Autodesk Inventor part; units mm, degrees
ref_plane "YZ Plane" through (0, 0, 0) normal (1, 0, 0) x (0, 1, 0)
ref_plane "XZ Plane" through (0, 0, 0) normal (0, 1, 0) x (-1, 0, 0)
ref_plane "XY Plane" through (0, 0, 0) normal (0, 0, 1) x (1, 0, 0)
sketch "Sketch1" plane through (0, 0, 0) normal (0, 0, 1) x (1, 0, 0)
  line L0 (-23.5242, 24.8428) -> (244.1465, 24.8428)
  line L1 (274.9258, 24.8428) -> (274.9258, -127.5572)
  line L2 (267.4299, -127.5572) -> (-29.8742, -127.5572)
  line L3 (-29.8742, -127.5572) -> (-29.8742, 18.4928)
  line L4 (250.4101, 19.5367) -> (273.6935, -120.1633)
  line L5 (-29.8742, -13.2572) -> (84.4258, -127.5572)
  arc A0 (-23.5242, 24.8428) -> (-29.8742, 18.4928) centre (-23.5242, 18.4928) ccw
  arc A1 (267.4299, -127.5572) -> (273.6935, -120.1633) centre (267.4299, -121.2072) ccw
  arc A2 (250.4101, 19.5367) -> (244.1465, 24.8428) centre (244.1465, 18.4928) ccw
  point P0 (-29.8742, 24.8428)
  point P1 (249.5258, 24.8428)
  dimension "d0" = 304.8
  dimension "d1" = 152.4
  dimension "d2" = 25.4
  dimension "d3" = 38.1
  dimension "d4" = 190.5
  dimension "d5" = 6.35
  dimension "d6" = 6.35
extrude "Extrusion1" add sketch "Sketch1" along normal blind 3.175 contours L0 A2 L4 A1 L2 L5 L3 A0
properties part number "FE-00004-09"
Read the model definition and answer for the solid it produces. Units are mm, in the model's axes. Give positions to 0.01 mm unless a question says otherwise; leave off trailing zeros. Write each loop counter-clockwise with the first axis right and the second up, starting at its lowest first coordinate (ties: lowest second). Pieces come first, ordered by that corner, then holes. Notation, with made-up numbers: (35.25, -20) - (45.25, -20) arc R6 ccw to (45.25, -13) - close; hole circle Ø7 at (45.5, -15). An arc over 180 degrees is marked (long way). Write item = value, one per line. Start each with the question number.
Item 1: Find the intervals of material crossed by probe 1 along X at (y, z) = (-88, 0.9); probe 2 along X at (y, z) = (-30, 0.35); probe 3 along Y at (x, z) = (-11.5, 1.3), in increasing order. Write a range as [from, to].
Item 2: Find section A-A (z = 2.65). Give the vertices of the cut face in (x, y), then the cut area to 3 significant figures.
Item 3: Find section C-C (x = 254). Give the vertices of the cut face in (y, z) (3 decimals).
Item 4: This flat-tipped pin is pushed along its axis until it touches: P1, Ø1.5, axis at x = 83.5, z = 1, coming from the -Y side. Where does it stop, or does it pass through?
Item 5: Find section B-B (y = -0.5). Give the vertices of the cut face in (x, z) (3 decimals), then the cut area to 3 significant figures.
Response:
q1.probe_1 = [44.87, 268.33]
q1.probe_2 = [-13.13, 258.67]
q1.probe_3 = [-31.63, 24.84]
q2.outline = (-29.87, -13.26) - (84.43, -127.56) - (267.43, -127.56) arc R6.35 ccw to (273.69, -120.16) - (250.41, 19.54) arc R6.35 ccw to (244.15, 24.84) - (-23.52, 24.84) arc R6.35 ccw to (-29.87, 18.49) - close
q2.area = 38,000 mm²
q3.outline = (-127.557, 0) - (-2.003, 0) - (-2.003, 3.175) - (-127.557, 3.175) - close
q4.P1 = -127.38
q5.outline = (-29.874, 0) - (253.75, 0) - (253.75, 3.175) - (-29.874, 3.175) - close
q5.area = 901 mm²
